Here's how the part is built. I have some questions about the finished solid (model axes, mm). A direction names the side the tool comes from. Coordinates: 2 decimals unless noted, no trailing zeros. Write each loop counter-clockwise with the first axis right and the second up, starting at its lowest first coordinate (ties: lowest second). Pieces come first, ordered by that corner, then holes. Notation, with made-up numbers: (12, -29) -> (39, -29) arc R28 cw to (39, -9) -> close; hole circle Ø5 at (70, 35.25). An arc over 180 degrees is marked (long way). Answer in a Markdown table with one row per item. Add a question column.
from build123d import *

# Parameters (mm, degrees)
SKETCH_1_W          = 50
SKETCH_1_H          = 50
EXTRUDE_1_DEPTH     = 25
SHELL_2_T           = 5
SKETCH_3_R          = 3.75
CUT_EXTRUDE_3_DEPTH = 17.5
FILLET_2_R          = 1
SKETCH_8_W          = 23
SKETCH_8_H          = 48
CUT_EXTRUDE_5_DEPTH = 5
SKETCH_2_R          = 3.125
CUT_EXTRUDE_6_DEPTH = 10
SKETCH_9_W          = 20.6
SKETCH_9_H          = 44
SKETCH_9_W_2        = 15
SKETCH_9_H_2        = 40
CUT_EXTRUDE_7_DEPTH = 40


with BuildPart() as part:
    # 草图1 → 凸台-拉伸1 (new body)
    with BuildSketch(Plane.XY):
        with Locations((25, 25)):
            Rectangle(SKETCH_1_W, SKETCH_1_H)
    extrude(amount=-EXTRUDE_1_DEPTH)

    # 抽壳2 (no face opened: a closed hollow body)
    add(offset(amount=-SHELL_2_T, mode=Mode.PRIVATE), mode=Mode.SUBTRACT)

    # 草图3 → 切除-拉伸3 (cut)
    with BuildSketch(Plane.ZY):
        with Locations((-12.488340482, 40.625)):
            Circle(SKETCH_3_R)
    extrude(amount=-CUT_EXTRUDE_3_DEPTH, mode=Mode.SUBTRACT)

    # 圆角2
    fillet_2_edges = [part.edges().sort_by_distance(p)[0] for p in [
        (50, 25, -25),
        (25, 50, -25),
        (0, 25, -25),
        (25, 50, 0),
        (50, 25, 0),
        (25, 0, 0),
        (0, 25, 0),
        (0, 50, -12.5),
        (50, 50, -12.5),
        (50, 0, -12.5),
        (0, 0, -12.5),
        (25, 0, -25),
    ]]
    fillet(fillet_2_edges, radius=FILLET_2_R)

    # 草图8 → 切除-拉伸5 (cut)
    with BuildSketch(Plane(origin=(50, 0, 0), x_dir=(0, 0, -1), z_dir=(1, 0, 0))):
        with Locations((12.5, 25)):
            Rectangle(SKETCH_8_W, SKETCH_8_H)
    extrude(amount=-CUT_EXTRUDE_5_DEPTH, mode=Mode.SUBTRACT)

    # 草图2 → 切除-拉伸6 (cut)
    with BuildSketch(Plane.ZY):
        with Locations((-19.5, 18.625)):
            Circle(SKETCH_2_R)
        with Locations((-19.5, 28)):
            Circle(SKETCH_2_R)
        with Locations((-5.5, 28)):
            Circle(SKETCH_2_R)
        with Locations((-5.5, 18.625)):
            Circle(SKETCH_2_R)
        with Locations((-12.5, 8.125)):
            Circle(SKETCH_2_R)
    extrude(amount=-CUT_EXTRUDE_6_DEPTH, mode=Mode.SUBTRACT)

    # 草图9 → 切除-拉伸7 (cut)
    with BuildSketch(Plane(origin=(45, 0, 0), x_dir=(0, 0, -1), z_dir=(1, 0, 0))):
        with Locations((12.5, 25)):
            Rectangle(SKETCH_9_W, SKETCH_9_H)
        with Locations((12.5, 25)):
            Rectangle(SKETCH_9_W_2, SKETCH_9_H_2, mode=Mode.SUBTRACT)
    extrude(amount=-CUT_EXTRUDE_7_DEPTH, mode=Mode.SUBTRACT)


solid = part.part
Q1. Imagine slicing it at B-B on x = 22. Please give me the cut outline in (y, z).
Q2. If we mould it in two halves opening along Y, with no side actions, what happens to faces 3 (the flat face through (25, 25, -25)), 4 (the flat face through (25, 0, -12)), 5 (the cylindrical face through (2.5, 31.1, -5.9))? For each: pulls with the +Y half, pulls with the -Y half, needs draft (parallel to the pull), parting line crosses it, or undercut.
Q3. Imagine slicing it at A-A on z = -5.5. Please give me the cut outline in (x, y) (3 decimals).
Q4. I need wall thicknesses on line 1 (Z direction, x = 2, y = 28) (3 decimals); line 2 (Y direction, x = 1.7, z = -19.5) (3 decimals); line 3 (Y direction, x = 2, z = -12.5). Which ranges of each line are inside material? Lowest first, please. Write a range as [from, to].
Q5. For faces 1 (the cylindrical face through (2.465, 21.723, -5.907)), 2 (the flat face through (25, 25, -2.2)), which set-ups out of +Z, -Z, +X, -X, +Y, -Y let a thin tool reach every point of the face, with its end or its side?
Q6. Imagine slicing it at D-D on z = -12.25. Please give me the cut outline in (x, y).
Q7. I'm going to push flat-ended pins straight in: P1, Ø1, axis at y = 23, z = -9, coming from the -X side; P2, Ø4, axis at y = 8.125, z = -12.5, coming from the -X side. Where does each tip first touch, or does it pass through?
Q8. Imagine slicing it at C-C on y = 33. Please give me the cut outline in (x, z), plus the area to 3 significant figures.
Result sheet:
| question | item | result |
|---|---|---|
| 1 | outline | (0, -24) arc R1 ccw to (1, -25) -> (49, -25) arc R1 ccw to (50, -24) -> (50, -1) arc R1 ccw to (49, 0) -> (1, 0) arc R1 ccw to (0, -1) -> close; hole (3, -22.8) -> (47, -22.8) -> (47, -2.2) -> (3, -2.2) -> close |
| 2 | face 3 | needs draft |
| 2 | face 4 | pulls with the -Y half |
| 2 | face 5 | undercut |
| 3 | outline | (0, 1) arc R1 ccw to (1, 0) -> (49, 0) arc R1 ccw to (50, 1) -> (45, 1) -> (45, 3) -> (5, 3) -> (5, 15.5) -> (0, 15.5) -> close; (0, 21.75) -> (5, 21.75) -> (5, 24.875) -> (0, 24.875) -> close; (0, 31.125) -> (5, 31.125) -> (5, 47) -> (45, 47) -> (45, 49) -> (50, 49) arc R1 ccw to (49, 50) -> (1, 50) arc R1 ccw to (0, 49) -> close |
| 4 | line 1 | z = [-25, -22.625], [-16.375, -8.625], [-2.375, 0] |
| 4 | line 2 | y = [0, 15.5], [21.75, 24.875], [31.125, 50] |
| 4 | line 3 | y = [0, 5], [11.25, 36.88], [44.37, 50] |
| 5 | face 1 | +X, -X |
| 5 | face 2 | +X |
| 6 | outline | (0, 1) arc R1 ccw to (1, 0) -> (49, 0) arc R1 ccw to (50, 1) -> (45, 1) -> (45, 3) -> (5, 3) -> (5, 5.01) -> (0, 5.01) -> close; (0, 11.24) -> (5, 11.24) -> (5, 36.88) -> (0, 36.88) -> close; (0, 44.37) -> (5, 44.37) -> (5, 47) -> (45, 47) -> (45, 49) -> (50, 49) arc R1 ccw to (49, 50) -> (1, 50) arc R1 ccw to (0, 49) -> close |
| 7 | P1 | stops at x = 0 |
| 7 | P2 | passes through |
| 8 | outline | (0, -24) arc R1 ccw to (1, -25) -> (49, -25) arc R1 ccw to (50, -24) -> (45, -24) -> (45, -22.8) -> (5, -22.8) -> (5, -2.2) -> (45, -2.2) -> (45, -1) -> (50, -1) arc R1 ccw to (49, 0) -> (1, 0) arc R1 ccw to (0, -1) -> close |
| 8 | area | 310 mm^2 |
